Source: CAD feature listing. Evaluate the final solid. Frame: model axes, mm. Face numbers are marked on the shaded views. A direction names the side the tool comes from. Give positions to 0.01 mm unless a question says otherwise; leave off trailing zeros. Write each loop counter-clockwise with the first axis right and the second up, starting at its lowest first coordinate (ties: lowest second). Pieces come first, ordered by that corner, then holes.
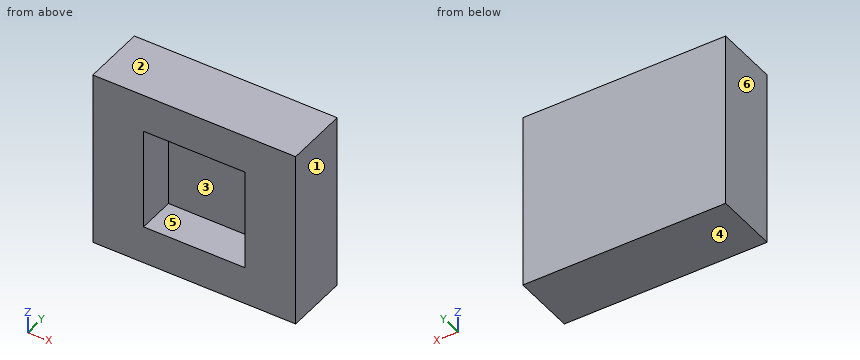
```python
from build123d import *

# Parameters (mm, degrees)
SKETCH1_W           = 10.16
SKETCH1_H           = 3.175
BOSS_EXTRUDE1_DEPTH = 4.445
SKETCH3_OUTSIDE_W   = 14.934
SKETCH3_OUTSIDE_H   = 13.664
SKETCH3_OUTSIDE_W_2 = 10.16
SKETCH3_OUTSIDE_H_2 = 8.89
SKETCH3_OUTSIDE_W_3 = 5.08
SKETCH3_OUTSIDE_H_3 = 5.08
CUT_EXTRUDE1_DEPTH  = 1.905


with BuildPart() as part:
    # Sketch1 → Boss-Extrude1 (new body, symmetric)
    with BuildSketch(Plane.XY):
        with Locations((0, -1.5875)):
            Rectangle(SKETCH1_W, SKETCH1_H)
    extrude(amount=BOSS_EXTRUDE1_DEPTH, both=True)

    # Sketch3 outside → Cut-Extrude1 (cut)
    with BuildSketch(Plane.XZ.offset(3.175)):
        Rectangle(SKETCH3_OUTSIDE_W, SKETCH3_OUTSIDE_H)
        Rectangle(SKETCH3_OUTSIDE_W_2, SKETCH3_OUTSIDE_H_2, mode=Mode.SUBTRACT)
        Rectangle(SKETCH3_OUTSIDE_W_3, SKETCH3_OUTSIDE_H_3)
    extrude(amount=-CUT_EXTRUDE1_DEPTH, mode=Mode.SUBTRACT)


solid = part.part
```
1. Section query B-B (z = 2). Return loops of the section in (x, y) (3 decimals), plus the area to 3 significant figures.
2. Section query C-C (x = -1.5). Return loops of the section in (y, z) (3 decimals).
3. Section query A-A (y = -1.95). Return loops of the section in (x, z) (3 decimals), plus the area to 3 significant figures.
4. Pull-direction query (Z, two-part tool) for the marked faces 1, 2, 3 and 4; classes: pulls with the +Z half, pulls with the -Z half, needs draft (parallel to the pull), parting line crosses it, or undercut.
5. Line query: probe 1 along X at (y, z) = (-2.95, 1.25); probe 2 along Z at (x, y) = (2.25, -1.65) (3 decimals); probe 3 along Y at (x, z) = (-1.25, 0.75). Output: solid intervals per line, ascending.
6. Access query for the marked faces 5 and 6. Directions: +Z, -Z, +X, -X, +Y, -Y. A direction counts if a zero-diameter tool reaches every point of the face in a straight line with its end or side. Return the directions, or none.
7. Pin query (flat end, axial travel): P1, Ø1.5, axis at x = -0.5, z = -0.5, coming from the -Y side. Return the tip coordinate at first contact, or that it passes through.
The answers:
1. outline: (-5.08, -3.175) - (-2.54, -3.175) - (-2.54, -1.27) - (2.54, -1.27) - (2.54, -3.175) - (5.08, -3.175) - (5.08, 0) - (-5.08, 0) - close
1. area: 22.6 mm2
2. outline: (-3.175, -4.445) - (0, -4.445) - (0, 4.445) - (-3.175, 4.445) - (-3.175, 2.54) - (-1.27, 2.54) - (-1.27, -2.54) - (-3.175, -2.54) - close
3. outline: (-5.08, -4.445) - (5.08, -4.445) - (5.08, 4.445) - (-5.08, 4.445) - close; hole (-2.54, -2.54) - (2.54, -2.54) - (2.54, 2.54) - (-2.54, 2.54) - close
3. area: 64.5 mm2
4. face 1: needs draft
4. face 2: pulls with the +Z half
4. face 3: undercut
4. face 4: pulls with the -Z half
5. probe 1: x = -5.08 to -2.54, 2.54 to 5.08
5. probe 2: z = -4.445 to -2.54, 2.54 to 4.445
5. probe 3: y = -1.27 to 0
6. face 5: -Y
6. face 6: +Z, -Z, -X, +Y, -Y
7. P1: stops at y = -1.27
